The figure shows three views and two pictorial views of one solid part (mm, origin at its lowest corner). Answer the questions. A direction names the side the tool comes from. Coordinates: 2 decimals unless noted, no trailing zeros. Order: outer loops, then holes, each group sorted by start corner. A loop starts at its lowest first (then second) coordinate and runs counter-clockwise, first axis right, second up. Notation, with made-up numbers: (76, 68) -> (122, 68) arc R23 ccw to (122, 88) -> close; hole circle Ø7 at (67.5, 38). An arc over 180 degrees is marked (long way). Return JSON: item names as keys, results as strings.
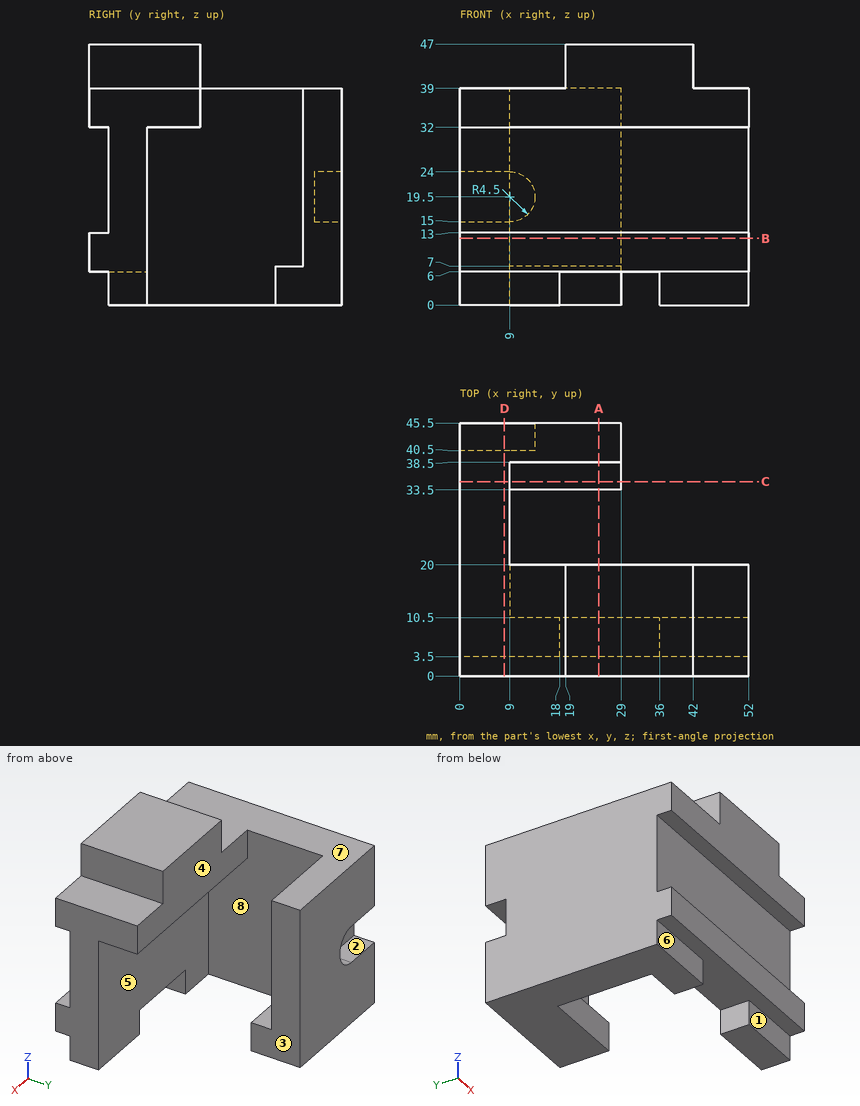
Item 1: The part is cut by section B-B on z = 12. Determine the outline of the cut face in (x, y), plus the area to 3 significant figures.
Answer list:
{"outline": "(0, 0) -> (52, 0) -> (52, 10.5) -> (9, 10.5) -> (9, 38.5) -> (29, 38.5) -> (29, 45.5) -> (0, 45.5) -> close", "area": "1,000 mm2"}
Item 2: Determine the mould class of the marked faces 6, 7 and 8 for opening direction Y: pulls with the +Y half, pulls with the -Y half, needs draft (parallel to the pull), parting line crosses it, or undercut.
Answer list:
{"face 6": "pulls with the -Y half", "face 7": "needs draft", "face 8": "undercut"}
Item 3: The part is cut by section A-A on x = 25. Determine the outline of the cut face in (y, z).
Answer list:
{"outline": "(0, 6) -> (10.5, 6) -> (10.5, 32) -> (20, 32) -> (20, 47) -> (0, 47) -> (0, 32) -> (3.5, 32) -> (3.5, 13) -> (0, 13) -> close; (33.5, 0) -> (45.5, 0) -> (45.5, 39) -> (38.5, 39) -> (38.5, 7) -> (33.5, 7) -> close"}
Item 4: The part is cut by section D-D on x = 8. Determine the outline of the cut face in (y, z), plus the area to 3 significant figures.
Answer list:
{"outline": "(0, 6) -> (3.5, 6) -> (3.5, 0) -> (45.5, 0) -> (45.5, 15) -> (40.5, 15) -> (40.5, 24) -> (45.5, 24) -> (45.5, 39) -> (0, 39) -> (0, 32) -> (3.5, 32) -> (3.5, 13) -> (0, 13) -> close", "area": "1,640 mm2"}
Item 5: Which of the six approach directions +Z, -Z, +X, -X, +Y, -Y give full straight-line access (tool end or side, diameter ignored) to the marked faces 1, 2, 3, 4 and 5?
Answer list:
{"face 1": "-Z, +X, -X, -Y", "face 2": "-X, +Y", "face 3": "+Z, -Z, +X, +Y", "face 4": "+Z, -Z, +X", "face 5": "-Z, +X"}
Item 6: The part is cut by section C-C on y = 35. Determine the outline of the cut face in (x, z), plus the area to 3 significant figures.
Answer list:
{"outline": "(0, 0) -> (29, 0) -> (29, 7) -> (9, 7) -> (9, 39) -> (0, 39) -> close", "area": "491 mm2"}
Item 7: Flat-ended cylindrical pins translate along their axes: pin 1 (3 mm diameter, centred on x = 7.5, z = 4, fed in from -Y); pin 2 (1 mm diameter, centred on x = 31.5, y = 2, fed in from -Z); pin 3 (1 mm diameter, centred on x = 23, y = 39.5, fed in from +Z). Find the tip coordinate at first contact, or state that the pin passes through.
Answer list:
{"pin 1": "y = 3.5", "pin 2": "z = 6", "pin 3": "z = 39"}
Item 8: Find the intervals of material crossed by probe 1 along Y at (x, z) = (25, 19.5); probe 2 along Y at (x, z) = (26.5, 38); probe 3 along Y at (x, z) = (38.5, 43), in increasing order.
Answer list:
{"probe 1": "3.5 to 10.5, 38.5 to 45.5", "probe 2": "0 to 20, 38.5 to 45.5", "probe 3": "0 to 20"}
